from build123d import *

# Parameters (mm, degrees)
SKETCH1_W             = 18
SKETCH1_H             = 3.175
BASE_DEPTH            = 3.175
SKETCH1_3_W           = 18
SKETCH1_3_H           = 3.175
RISER_DEPTH           = 66.675
F_6_CLEARANCE_HOLE2_D = 3.7973
F_6_CLEARANCE_HOLE1_D = 3.7973
FILLET1_R             = 10
FILLET2_R             = 9
FILLET3_R             = 10
FILLET4_R             = 1.27


with BuildPart() as part:
    # Sketch1 → Base (new body)
    with BuildSketch(Plane(origin=(0, 0, 0), x_dir=(1, 0, 0), z_dir=(0, 1, 0))):
        with BuildLine():
            Line((-9, 0), (-9, 20))
            Line((-9, 20), (9, 20))
            Line((9, 20), (9, 0))
            ThreePointArc((9, 0), (0, -9), (-9, 0))
        make_face()
        with Locations((0, 21.5875)):
            Rectangle(SKETCH1_W, SKETCH1_H)
    extrude(amount=-BASE_DEPTH)

    # Sketch1<3> → Riser (add)
    with BuildSketch(Plane(origin=(0, 0, 0), x_dir=(1, 0, 0), z_dir=(0, 1, 0))):
        with Locations((0, 21.5875)):
            Rectangle(SKETCH1_3_W, SKETCH1_3_H)
    extrude(amount=RISER_DEPTH)

    # #6 Clearance Hole2 (through all)
    with Locations(Plane(origin=(0, 0, 0), x_dir=(-1, 0, 0), z_dir=(0, 1, 0))):
        with Locations((0, 0)):
            Hole(F_6_CLEARANCE_HOLE2_D / 2)

    # #6 Clearance Hole1 (through all)
    with Locations(Plane.XY.offset(-20)):
        with Locations((0, 59.575), (0, 28.575)):
            Hole(F_6_CLEARANCE_HOLE1_D / 2)

    # Fillet1
    fillet1_edges = [part.edges().sort_by_distance(p)[0] for p in [
        (0, 0, -20),
    ]]
    fillet(fillet1_edges, radius=FILLET1_R)

    # Fillet2
    fillet2_edges = [part.edges().sort_by_distance(p)[0] for p in [
        (-9, 66.675, -21.5875),
        (9, 66.675, -21.5875),
    ]]
    fillet(fillet2_edges, radius=FILLET2_R - 0.0001)  # a hair under: the kernel refuses the full size

    # Fillet3
    fillet3_edges = [part.edges().sort_by_distance(p)[0] for p in [
        (0, -3.175, -23.175),
    ]]
    fillet(fillet3_edges, radius=FILLET3_R)

    # Fillet4
    fillet4_edges = [part.edges().sort_by_distance(p)[0] for p in [
        (0, -3.175, 9),
        (9, -3.175, -6.5875),
        (-9, -3.175, -6.5875),
        (9, 2.928932188, -17.071067812),
        (-9, 2.928932188, -17.071067812),
        (-9, 33.83755, -20),
        (6.36399032, 64.03899032, -23.175),
        (-6.36399032, 64.03899032, -23.175),
        (9, 33.83755, -20),
        (6.36399032, 64.03899032, -20),
        (-6.36399032, 64.03899032, -20),
        (9, 0, -5),
        (9, 32.25005, -23.175),
        (9, -0.246067812, -20.246067812),
        (-9, 32.25005, -23.175),
        (-9, -0.246067812, -20.246067812),
        (0, 0, 9),
        (-9, 0, -5),
    ]]
    fillet(fillet4_edges, radius=FILLET4_R)


solid = part.part
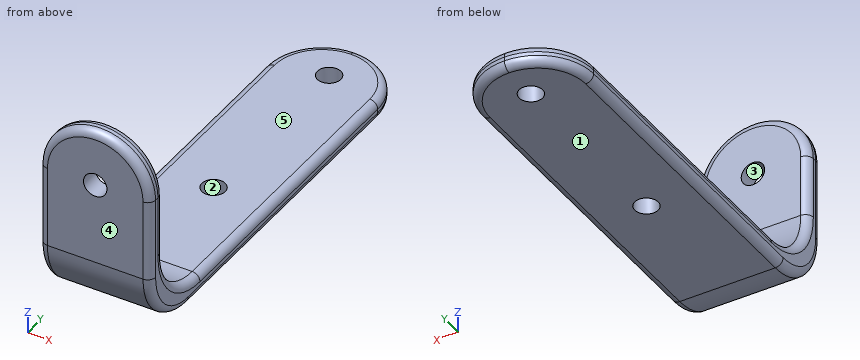
Geometry check sheet. Reference: the model listing, model coordinates, mm. Face numbers are marked on the shaded views. A direction names the side the tool comes from. Give positions to 0.01 mm unless a question says otherwise; leave off trailing zeros. Loops run counter-clockwise (first coordinate to the right, second up) from the corner with the lowest first, then second, coordinate; pieces in that order, holes last.
(1) Section check C-C on x = 1. Count the separate pieces of the cut face and the enclosed holes in it, then the cut area to 3 significant figures.
From the geometry:
separate pieces: 4
enclosed holes: 0
area: 281 mm2
(2) Depth check by flat-ended pin: pin 1 Ø7.5 at (x, z) = (-3, -2) entering from +Y; pin 2 Ø10 at (y, z) = (42, -16) entering from +X; pin 3 Ø1.5 at (x, y) = (-1, 46) entering from +Z. Enter the tip coordinate at first touch or a pass-through.
From the geometry:
pin 1: stops at y = 0
pin 2: stops at x = 8.97
pin 3: stops at z = -20
(3) Release check for a two-part mould opening along Z. For the marked faces 1, 2 and 3 record: released by +Z, released by -Z, zero draft, split by the parting line, or undercut.
From the geometry:
face 1: released by -Z
face 2: zero draft
face 3: undercut
(4) Section check B-B on y = 41.5. Record the cut outline in (x, z) (3 decimals).
From the geometry:
outline: (-9, -21.905) arc R1.27 ccw to (-7.73, -23.175) - (7.73, -23.175) arc R1.27 ccw to (9, -21.905) - (9, -21.27) arc R1.27 ccw to (7.73, -20) - (-7.73, -20) arc R1.27 ccw to (-9, -21.27) - close
(5) Section check A-A on z = -3.5. Record the cut outline in (x, y) (3 decimals).
From the geometry:
outline: (-9, -1.905) arc R1.27 ccw to (-7.73, -3.175) - (7.73, -3.175) arc R1.27 ccw to (9, -1.905) - (9, -1.27) arc R1.27 ccw to (7.73, 0) - (-7.73, 0) arc R1.27 ccw to (-9, -1.27) - close
(6) Set-up check for the marked faces 4 and 5: record each of +Z, -Z, +X, -X, +Y, -Y from which the full face is reachable in a straight line by a thin tool's end or side.
From the geometry:
face 4: +Z, -Z, +X, -X, -Y
face 5: +Z, +X, -X, +Y
(7) Thickness scan on L1, parallel to Y at x = 0, z = -21.3 (3 decimals); L2, parallel to Z at x = -1, y = 16.5 (3 decimals); L3, parallel to Y at x = -4.75, z = 5.5 (3 decimals). Record the ranges inside material, lowest first.
From the geometry:
L1: y = 0.995 to 26.676, 30.474 to 57.676, 61.474 to 66.675
L2: z = -23.175 to -20
L3: y = -3.175 to 0
